Study the drawing (mm; zero at the part's minimum x, y, z) and answer. Give positions to 0.01 mm unless a question says otherwise; leave off trailing zeros. Order: outer loops, then holes, each group sorted by start corner. A loop starts at its lowest first (then second) coordinate and runs counter-clockwise, first axis right, second up. Notation, with made-up numbers: (-33, 28) - (0, 28) arc R21 ccw to (0, 47) - close; hole circle Ø10 at (61, 10.25). An arc over 180 degrees is marked (long way). Return JSON: item names as keys, results as strings.
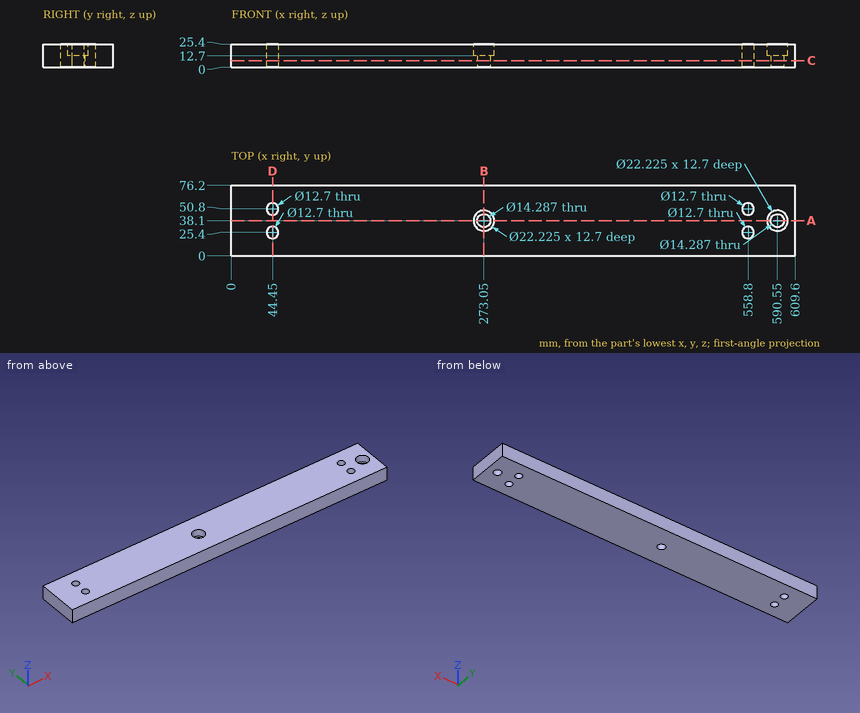
Q1. A cutting plane is placed at D-D (x = 44.45). Write down the section's boundary in (y, z), and give its area (3 significant figures).
Values:
{"outline": "(0, 0) - (19.05, 0) - (19.05, 25.4) - (0, 25.4) - close; (31.75, 0) - (44.45, 0) - (44.45, 25.4) - (31.75, 25.4) - close; (57.15, 0) - (76.2, 0) - (76.2, 25.4) - (57.15, 25.4) - close", "area": "1,290 mm²"}
Q2. A cutting plane is placed at C-C (z = 7.5). Write down the section's boundary in (x, y).
Values:
{"outline": "(0, 0) - (609.6, 0) - (609.6, 76.2) - (0, 76.2) - close; hole circle Ø12.7 at (44.45, 25.4); hole circle Ø12.7 at (44.45, 50.8); hole circle Ø14.29 at (273.05, 38.1); hole circle Ø12.7 at (558.8, 25.4); hole circle Ø12.7 at (558.8, 50.8); hole circle Ø14.29 at (590.55, 38.1)"}
Q3. A cutting plane is placed at B-B (x = 273.05). Write down the section's boundary in (y, z).
Values:
{"outline": "(0, 0) - (30.96, 0) - (30.96, 12.7) - (26.99, 12.7) - (26.99, 25.4) - (0, 25.4) - close; (45.24, 0) - (76.2, 0) - (76.2, 25.4) - (49.21, 25.4) - (49.21, 12.7) - (45.24, 12.7) - close"}
Q4. Given pin 1 (6.5 mm diameter, centred on x = 594, y = 34.5, fed in from +Z); pin 2 (11.5 mm diameter, centred on x = 44.45, y = 50.8, fed in from +Z), each flat-ended and moving along its own axis, determine where each tip first touches the part or whether it passes through.
Values:
{"pin 1": "stops at z = 12.7", "pin 2": "passes through"}
Q5. Consider L1, parallel to X at y = 25.5, z = 6.5; L2, parallel to X at y = 26.5, z = 19 (1 decimal); L3, parallel to Y at x = 558.8, z = 13. Determine where each line is inside the solid, lowest interval first.
Values:
{"L1": "x = 0 to 38.1, 50.8 to 552.45, 565.15 to 609.6", "L2": "x = 0 to 38.2, 50.7 to 552.5, 565.1 to 609.6", "L3": "y = 0 to 19.05, 31.75 to 44.45, 57.15 to 76.2"}
Q6. A cutting plane is placed at A-A (y = 38.1). Write down the section's boundary in (x, z).
Values:
{"outline": "(0, 0) - (265.91, 0) - (265.91, 12.7) - (261.94, 12.7) - (261.94, 25.4) - (0, 25.4) - close; (280.19, 0) - (583.41, 0) - (583.41, 12.7) - (579.44, 12.7) - (579.44, 25.4) - (284.16, 25.4) - (284.16, 12.7) - (280.19, 12.7) - close; (597.69, 0) - (609.6, 0) - (609.6, 25.4) - (601.66, 25.4) - (601.66, 12.7) - (597.69, 12.7) - close"}
